Autodesk Inventor part; units mm, degrees
ref_plane "YZ Plane" through (0, 0, 0) normal (1, 0, 0) x (0, 1, 0)
ref_plane "XZ Plane" through (0, 0, 0) normal (0, 1, 0) x (-1, 0, 0)
ref_plane "XY Plane" through (0, 0, 0) normal (0, 0, 1) x (1, 0, 0)
sketch "Sketch1" plane through (0, 0, 0) normal (0, 1, 0) x (-1, 0, 0)
  line L0 (7.5, 6.6144) -> (7.5, -6.6144)
  line L1 (-7.5, -6.6144) -> (-7.5, 6.6144)
  arc A0 (-7.5, -6.6144) -> (7.5, -6.6144) centre (0, 0) ccw
  arc A1 (7.5, 6.6144) -> (-7.5, 6.6144) centre (0, 0) ccw
  dimension "d1" = 15
  dimension "d2" = 7.5
  dimension "d3" = 10
  dimension "d4" = 10
extrude "Extrusion1" add sketch "Sketch1" along normal blind 25
sketch "Sketch2" plane through (0, 0, 0) normal (0, -1, 0) x (1, 0, 0)
  circle A0 centre (0, 0) radius 3
  dimension "d7" = 6
extrude "Extrusion2" add sketch "Sketch2" along normal blind 2
sketch "Sketch3" plane through (0, -2, 0) normal (0, -1, 0) x (1, 0, 0)
  circle A0 centre (0, 0) radius 2
  dimension "d10" = 4
extrude "Extrusion3" add sketch "Sketch3" along normal blind 3
sketch "Sketch4" plane through (0, 25, 0) normal (0, 1, 0) x (1, 0, 0)
  circle A0 centre (0, 0) radius 2
  circle A1 centre (0, 0) radius 5
  dimension "d13" = 10
extrude "Extrusion4" add sketch "Sketch4" along normal blind 3 contours A0 | A1
sketch "Sketch5" plane through (7.5, 0, 6.6144) normal (1, 0, 0) x (0, 0, -1)
  line L0 (0, 0) -> (0, 25)
  line L1 (13.2288, 0) -> (13.2288, 25)
  line L2 (0, 25) -> (13.2288, 25)
  line L3 (13.2288, 25) -> (13.2288, 18)
  line L4 (13.2288, 18) -> (0, 18)
  line L5 (0, 18) -> (0, 25)
  point P0 (6.6144, 0)
  point P1 (0, 18)
  dimension "d16" = 7
extrude "Extrusion5" add sketch "Sketch5" along normal blind 4
sketch "Sketch7" plane through (0, -5, 0) normal (0, -1, 0) x (1, 0, 0)
  circle A0 centre (0, 0) radius 2.5
  dimension "d21" = 5
extrude "Extrusion7" add sketch "Sketch7" along normal blind 4
sketch "Sketch8" plane through (0, -9, 0) normal (0, -1, 0) x (1, 0, 0)
  circle A0 centre (0, 0) radius 1.5
  circle A1 centre (0, 0) radius 2.5
  line L0 (-0.5, 1) -> (0.5, 1)
  line L1 (0.5, 1) -> (0.5, 2)
  line L2 (0.5, 2) -> (-0.5, 2) construction
  line L3 (-0.5, 2) -> (-0.5, 1)
  line L4 (-0.5, 1) -> (0.5, 2) construction
  line L5 (0.5, 1) -> (-0.5, 2) construction
  circle A2 centre (0, 2) radius 0.5
  line L6 (-0.3536, 1.0607) -> (-1.0607, 1.7678)
  line L7 (-1.0607, 1.7678) -> (-1.7678, 1.0607) construction
  line L8 (-1.0607, 0.3536) -> (-1.0607, 1.7678) construction
  circle A3 centre (-1.4142, 1.4142) radius 0.5
  line L9 (-1.7678, 1.0607) -> (-1.0607, 0.3536)
  line L10 (-1, 0.5) -> (-2, 0.5)
  line L11 (-2, 0.5) -> (-2, -0.5) construction
  line L12 (-1, -0.5) -> (-2, 0.5) construction
  circle A4 centre (-2, 0) radius 0.5
  line L13 (-2, -0.5) -> (-1, -0.5)
  line L14 (-1.0607, -0.3536) -> (-1.7678, -1.0607)
  line L15 (-1.7678, -1.0607) -> (-1.0607, -1.7678) construction
  line L16 (-0.3536, -1.0607) -> (-1.7678, -1.0607) construction
  circle A5 centre (-1.4142, -1.4142) radius 0.5
  line L17 (-1.0607, -1.7678) -> (-0.3536, -1.0607)
  line L18 (-0.5, -1) -> (-0.5, -2)
  line L19 (-0.5, -2) -> (0.5, -2) construction
  line L20 (0.5, -1) -> (-0.5, -2) construction
  circle A6 centre (0, -2) radius 0.5
  line L21 (0.5, -2) -> (0.5, -1)
  line L22 (0.3536, -1.0607) -> (1.0607, -1.7678)
  line L23 (1.0607, -1.7678) -> (1.7678, -1.0607) construction
  line L24 (1.0607, -0.3536) -> (1.0607, -1.7678) construction
  circle A7 centre (1.4142, -1.4142) radius 0.5
  line L25 (1.7678, -1.0607) -> (1.0607, -0.3536)
  line L26 (1, -0.5) -> (2, -0.5)
  line L27 (2, -0.5) -> (2, 0.5) construction
  line L28 (1, 0.5) -> (2, -0.5) construction
  circle A8 centre (2, 0) radius 0.5
  line L29 (2, 0.5) -> (1, 0.5)
  line L30 (1.0607, 0.3536) -> (1.7678, 1.0607)
  line L31 (1.7678, 1.0607) -> (1.0607, 1.7678) construction
  line L32 (0.3536, 1.0607) -> (1.7678, 1.0607) construction
  circle A9 centre (1.4142, 1.4142) radius 0.5
  line L33 (1.0607, 1.7678) -> (0.3536, 1.0607)
  point P0 (0, 1.5)
  point P1 (-1.0607, 1.0607)
  point P2 (-1.5, 0)
  point P3 (-1.0607, -1.0607)
  point P4 (0, -1.5)
  point P5 (1.0607, -1.0607)
  point P6 (1.3536, -0.6464)
  point P7 (1.7678, -1.7678)
  point P8 (0, 2.5)
  point P9 (0.5, 1.4142)
  point P10 (1.0607, -1.7678)
  point P11 (0.6464, -1.3536)
  point P12 (0.5, -1.4142)
  point P13 (0, -2.5)
  point P14 (-0.5, -1.4142)
  point P15 (-0.6464, -1.3536)
  point P16 (-1.7678, -1.7678)
  point P17 (-1.7678, -1.0607)
  point P18 (-1.3536, -0.6464)
  point P19 (-1.4142, -0.5)
  point P20 (-2.5, 0)
  point P21 (-1.4142, 0.5)
  point P22 (-1.3536, 0.6464)
  point P23 (-1.7678, 1.7678)
  point P24 (-0.6464, 1.3536)
  point P25 (-0.5, 1.4142)
  point P26 (1.5, 0)
  point P27 (1.0607, 1.0607)
  point P28 (0.6464, 1.3536)
  point P29 (1.7678, 1.7678)
  point P30 (1.3536, 0.6464)
  point P31 (1.4142, 0.5)
  point P32 (2.5, 0)
  point P33 (1.4142, -0.5)
  dimension "d24" = 3
  dimension "d25" = 5
  dimension "d26" = 1
  dimension "d29" = 360
extrude "Extrusion8" cut sketch "Sketch8" against normal blind 4 contours A0 L30 A9 A1 A8 L29 | L26 A8 A1 A7 L25 A0 | A9 L33 A0 L1 A2 A1 | A1 A6 L21 A0 L22 A7 | A2 L3 A0 L6 A3 A1 | A1 A5 L17 A0 L18 A6 | A3 L9 A0 L10 A4 A1 | A1 A4 L13 A0 L14 A5
sketch "Sketch9" plane through (0, -9, 0) normal (0, -1, 0) x (1, 0, 0)
  circle A0 centre (0, 0) radius 1
  dimension "d33" = 2
extrude "Extrusion9" add sketch "Sketch9" along normal blind 1
fillet "Fillet1" radius 0.25 1 edges at (-1, -10, 0)
sketch "Sketch10" plane through (0, 25, 0) normal (0, 1, 0) x (1, 0, 0)
  circle A0 centre (9.5, 4.6144) radius 1
  circle A1 centre (9.5, -4.6144) radius 1
  line L0 (11.5, 6.6144) -> (11.5, -6.6144)
  line L1 (7.5, 6.6144) -> (11.5, 6.6144)
  line L2 (7.5, -6.6144) -> (11.5, -6.6144)
  point P0 (0, 0)
  dimension "d37" = 2
  dimension "d38" = 2
  dimension "d39" = 2
  dimension "d40" = 2
  dimension "d41" = 2
  dimension "d42" = 2
extrude "Extrusion10" add sketch "Sketch10" along normal blind 6
properties part number "motor"
Input: part model. Units: mm. Frame: model coordinates. A direction names the side the tool comes from. Coordinates: 2 decimals unless noted, no trailing zeros. Order: outer loops, then holes, each group sorted by start corner. A loop starts at its lowest first (then second) coordinate and runs counter-clockwise, first axis right, second up. Notation, with made-up numbers: (75, -29) - (106, -29) arc R30 ccw to (106, 0) - close; hole circle Ø4 at (63, 86.25). An arc over 180 degrees is marked (long way). Return JSON: item names as keys, results as strings.
Q1. First-contact query: pin 1 (1 mm diameter, centred on x = -4, y = 0, fed in from -Z); pin 2 (1.2 mm diameter, centred on x = 8.5, y = 20, fed in from -Z); pin 3 (0.6 mm diameter, centred on x = 0, z = -2, fed in from +Y). Flat tips, straight axial feed; report the tip coordinate or a pass-through.
The answers:
{"pin 1": "stops at z = -9.37", "pin 2": "stops at z = -6.61", "pin 3": "stops at y = 28"}
Q2. Access query for faces 4 (the flat face through (9, 21, -6.614)), 5 (the flat face through (0, 28, 0)), 6 (the cylindrical face through (-1.775, -7.028, -1.76)), 7 (the flat face through (7.5, 9, 0)). Directions: +Z, -Z, +X, -X, +Y, -Y. A direction counts if a zero-diameter tool reaches every point of the face in a straight line with its end or side. Return the directions, or none.
The answers:
{"face 4": "-Z, +X, +Y, -Y", "face 5": "+Z, -Z, -X, +Y", "face 6": "-Y", "face 7": "+Z, -Z, +X, -Y"}
Q3. Cut plane A-A (x = 9.5). Return loops of the section in (y, z).
The answers:
{"outline": "(18, -6.61) - (25, -6.61) - (25, -5.61) - (31, -5.61) - (31, -3.61) - (25, -3.61) - (25, 3.61) - (31, 3.61) - (31, 5.61) - (25, 5.61) - (25, 6.61) - (18, 6.61) - close"}
Q4. Cut plane D-D (x = 0). Return loops of the section in (y, z), then the cut area to 3 significant figures.
The answers:
{"outline": "(-10, -0.75) arc R0.25 ccw to (-9.75, -1) - (-9, -1) - (-9, -2.5) - (-5, -2.5) - (-5, -2) - (-2, -2) - (-2, -3) - (0, -3) - (0, -10) - (25, -10) - (25, -5) - (28, -5) - (28, 5) - (25, 5) - (25, 10) - (0, 10) - (0, 3) - (-2, 3) - (-2, 2) - (-5, 2) - (-5, 2.5) - (-9, 2.5) - (-9, 1) - (-9.75, 1) arc R0.25 ccw to (-10, 0.75) - close", "area": "576 mm2"}
Q5. Cut plane B-B (y = 22). Return loops of the section in (x, z).
The answers:
{"outline": "(-7.5, -6.61) arc R10 ccw to (7.5, -6.61) - (11.5, -6.61) - (11.5, 6.61) - (7.5, 6.61) arc R10 ccw to (-7.5, 6.61) - close"}
Q6. Ray query, probe 1 along Y at (x, z) = (2, -7); probe 2 along Z at (x, y) = (8.25, 23.5); probe 3 along Y at (x, z) = (2, -2.5). Return the intervals inside material, ascending.
The answers:
{"probe 1": "y = 0 to 25", "probe 2": "z = -6.61 to 6.61", "probe 3": "y = 0 to 28"}
Q7. Cut plane C-C (z = -8.25). Return loops of the section in (x, y), then the cut area to 3 significant figures.
The answers:
{"outline": "(-5.65, 0) - (5.65, 0) - (5.65, 25) - (-5.65, 25) - close", "area": "283 mm2"}
Q8. Draft query along Z for faces 1 (the flat face through (9, 31, -5)), 2 (the cylindrical face through (-2.5, -7, 0)), 3 (the cylindrical face through (1.76, -7.028, -1.775)). Return one class per face: +Z half, -Z half, draft (parallel to the pull), parting line (faces both ways), or undercut.
The answers:
{"face 1": "draft", "face 2": "parting line", "face 3": "undercut"}
